Design review of the part built by this model. Coordinates are the model's own, in mm. A direction names the side the tool comes from. Coordinates: 2 decimals unless noted, no trailing zeros. Loops run counter-clockwise (first coordinate to the right, second up) from the corner with the lowest first, then second, coordinate; pieces in that order, holes last. Notation, with made-up numbers: (56, -19.5) - (62, -19.5) arc R37 cw to (62, 19.5) - close; hole circle Ø1 at (67.25, 58.25). An arc over 180 degrees is marked (long way). Use one line per item in the form item = value. Start each with the question number.
(1) Tool access review of faces 1 (the face through (9.84, 15.43, 16.22)), 2 (the face through (12.27, 23.6, 51.72)), 3 (the face through (0, -25, 12)): name each direction out of +Z, -Z, +X, -X, +Y, -Y from which nothing blocks a thin tool from reaching the whole face with its end or side.
(2) Add section B-B (z = 28.5). State the section outline as (x, y) points.
(3) Add section A-A (z = 65.5). State the section outline as (x, y) points, plus the area to 3 significant figures.
(4) For L1, parallel to X at y = 0, z = 41; L2, parallel to Y at x = 0, z = 14, list the stretches that pass through material, from the lowest coordinate up.
(5) The part is to be moulded in two halves that separate along X. For faces 4 (the face through (-6.94, 31.24, 29.46)), 5 (the face through (5, 18, 32)), 6 (the face through (0, 25, 11)), say which applies: pulls with the +X half, pulls with the -X half, needs draft (parallel to the pull), parting line crosses it, or undercut.
(6) Clearance check with flat-ended pins moving along their axes: pin 1 Ø8 at (y, z) = (-1.5, 25) entering from +X; pin 2 Ø5 at (x, z) = (24.5, 48) entering from -Y; pin 3 Ø3 at (x, z) = (0, 10.5) entering from -Y; pin 4 Ø8 at (x, z) = (12, 33.5) entering from +Y. State where each tip first meets the part, or that it passes through.
Autodesk Fusion 360 part; units mm, degrees
sketch "Sketch1" plane through (0, 0, 0) normal (0, 0, 1) x (1, 0, 0)
  circle A0 centre (0, 0) radius 24.5
  circle A1 centre (0, 0) radius 18.3
  dimension "d1" = 49
  dimension "d7" = 36.6
ref_plane "WorkPlane1" through (0, 0, 27) normal (0, 0, 1) x (1, 0, 0)
sketch "Sketch2" plane through (0, 0, 27) normal (0, 0, 1) x (1, 0, 0)
  circle A0 centre (0, 0) radius 25
  circle A1 centre (0, 0) radius 18.3
  dimension "d6" = 50
  dimension "d8" = 36.6
loft "Loft3" add profiles "Sketch1", "Sketch2" section 1 section 2
loft "Loft4" cut profiles "Sketch1", "Sketch2" section 1 contours A1 section 2 contours A1
sketch "Sketch3" plane through (0, 0, 27) normal (0, 0, 1) x (1, 0, 0)
  circle A0 centre (0, 0) radius 32
  circle A1 centre (0, 0) radius 26.6
  circle A2 centre (0, 0) radius 24.1
  dimension "d9" = 64
  dimension "d10" = 53.2
  dimension "d15" = 48.2
extrude "Extrude1" add sketch "Sketch2" sketch "Sketch3" along normal blind 5 of sketch 2 contours A0 | A1
extrude "Extrude2" add sketch "Sketch3" along normal blind 45 contours A1
sketch "Sketch5" plane through (0, 0, 0) normal (0, 1, 0) x (1, 0, 0)
  ellipse E0 centre (0, -11.5) end of major axis (6, -11.5) minor radius 3.75
  line L0 (-6, -11.5) -> (6, -11.5)
  line L1 (0, -15.25) -> (0, -7.75)
  line L2 (-32, -27) -> (32, -27)
  dimension "d20" = 12
  dimension "d21" = 7.5
  dimension "d23" = 15.5
extrude "Extrude4" add sketch "Sketch5" along normal blind 2 from surface at 23
extrude "Extrude5" add sketch "Sketch5" against normal blind 2 from surface at -23
fillet "Fillet1" radius 1 2 edges at (-6, 25, 11.5) (-6, -25, 11.5)
Computed values:
q1.face_1 = +Z, -Z
q1.face_2 = +Z
q1.face_3 = -Z, +X, -X, -Y
q2.outline = circle Ø64 at (0, 0); hole circle Ø36.6 at (0, 0)
q3.outline = circle Ø53.2 at (0, 0); hole circle Ø48.2 at (0, 0)
q3.area = 398 mm^2
q4.L1 = -26.6 to -24.1, 24.1 to 26.6
q4.L2 = -25 to -18.3, 18.3 to 25
q5.face_4 = parting line crosses it
q5.face_5 = undercut
q5.face_6 = needs draft
q6.pin_1 = 32
q6.pin_2 = -14.95
q6.pin_3 = -25
q6.pin_4 = 30.91
